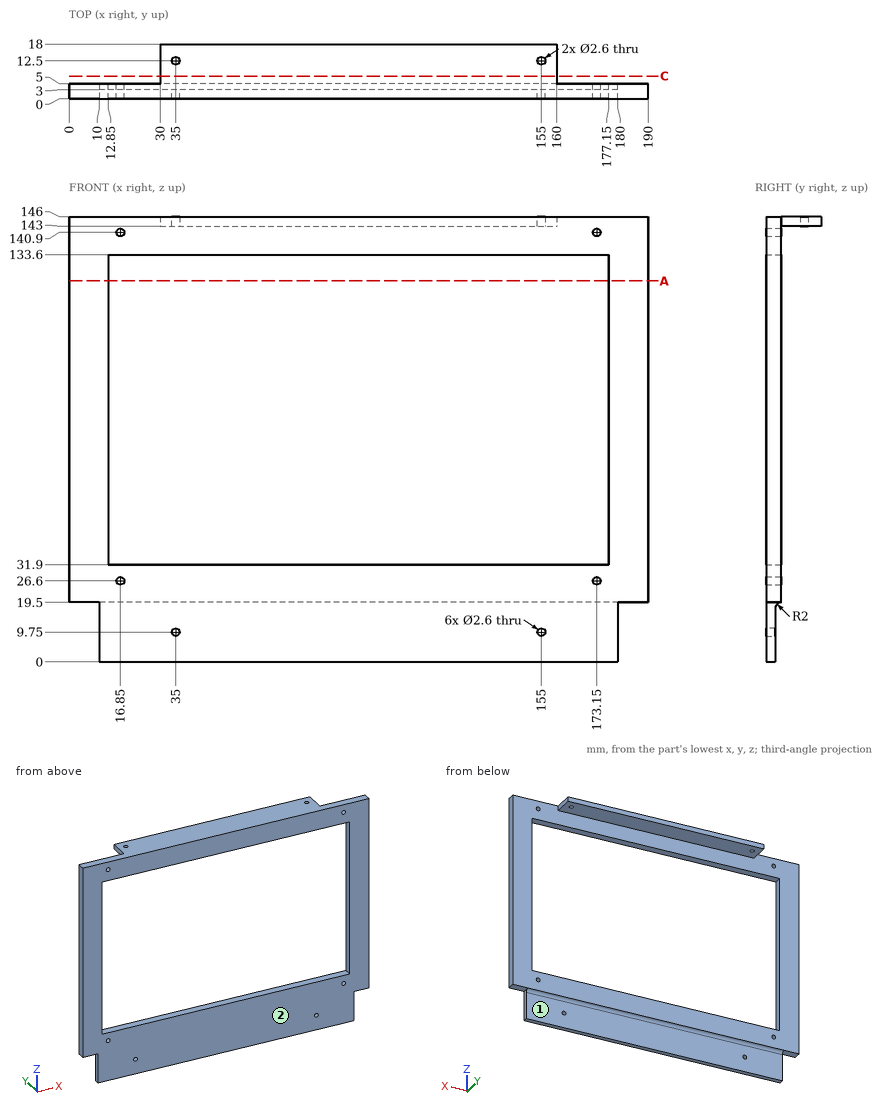
Design review of the part shown in the three views and the two pictorial views. Dimensions are in mm from the part's minimum x, y and z. A direction names the side the tool comes from. Coordinates: 2 decimals unless noted, no trailing zeros. Loops run counter-clockwise (first coordinate to the right, second up) from the corner with the lowest first, then second, coordinate; pieces in that order, holes last.
Q1. We need section A-A on z = 125. State the section outline as (x, y) points, and give its area (4 significant figures).
Reported:
outline: (0, 0) - (12.85, 0) - (12.85, 5) - (0, 5) - close; (177.15, 0) - (190, 0) - (190, 5) - (177.15, 5) - close
area: 128.5 mm2
Q2. For pin 1 (4 mm diameter, centred on x = 16.85, z = 26.6, fed in from +Y); pin 2 (3 mm diameter, centred on x = 35, z = 9.75, fed in from +Y); pin 3 (1.6 mm diameter, centred on x = 155, y = 12.5, fed in from -Z); pin 4 (3 mm diameter, centred on x = 34, y = 5.5, fed in from -Z), all flat-tipped, find the tip position at first contact; note any pin that passes through.
Reported:
pin 1: stops at y = 5
pin 2: stops at y = 3
pin 3: passes through
pin 4: stops at z = 19.23
Q3. To check wall thickness, follow line 1 (Z direction, x = 173.15, y = 1.35); line 2 (Z direction, x = 35, y = 2.15); line 3 (X direction, y = 1.45, z = 140.9). State the ranges of each line that lie inside material, in increasing order.
Reported:
line 1: z = 0 to 25.3, 27.9 to 31.9, 133.6 to 139.6, 142.2 to 146
line 2: z = 0 to 8.45, 11.05 to 31.9, 133.6 to 146
line 3: x = 0 to 15.55, 18.15 to 171.85, 174.45 to 190
Q4. We need section C-C on y = 7.5. State the section outline as (x, z) points, and give its area (3 significant figures).
Reported:
outline: (30, 143) - (160, 143) - (160, 146) - (30, 146) - close
area: 390 mm2
Q5. Tool access review of the marked faces 1 and 2: name each direction out of +Z, -Z, +X, -X, +Y, -Y from which nothing blocks a thin tool from reaching the whole face with its end or side.
Reported:
face 1: -Z, +X, -X, +Y
face 2: +Z, -Z, +X, -X, -Y
